The listing builds one solid part. Answer for the finished solid, in the listing's coordinates (mm). Coordinates: 2 decimals unless noted, no trailing zeros. Loops run counter-clockwise (first coordinate to the right, second up) from the corner with the lowest first, then second, coordinate; pieces in that order, holes last. Notation, with made-up numbers: M 52,61 L 75,61 A24 ccw 75,79 Z; hole C -33.75,-5.75 d3. An arc over 180 degrees is marked long. Answer as CSV lines item,"result". Start each with the question number.
```python
from build123d import *

# Parameters (mm, degrees)
SKETCH1_R                = 6.35
SKETCH1_R_2              = 2.159
BOSS_EXTRUDE1_DEPTH      = 5.0038
SKETCH6_R                = 9.715843696
SKETCH6_R_2              = 2.159
BOSS_EXTRUDE3_DEPTH      = 0.254
BOSS_EXTRUDE3_DEPTH_BACK = 5.0038
SKETCH2_R                = 2.159
CUT_EXTRUDE1_DEPTH       = 19.812


with BuildPart() as part:
    # Sketch1 → Boss-Extrude1 (new body)
    with BuildSketch(Plane.XY):
        with BuildLine():
            Line((-101.6, 12.7), (127, 12.7))
            ThreePointArc((127, 12.7), (139.7, 0), (127, -12.7))
            Line((127, -12.7), (-101.6, -12.7))
            ThreePointArc((-101.6, -12.7), (-114.3, 0), (-101.6, 12.7))
        make_face()
        with Locations((127, 0)):
            Circle(SKETCH1_R, mode=Mode.SUBTRACT)
        with Locations((-101.6, 0)):
            Circle(SKETCH1_R_2, mode=Mode.SUBTRACT)
    extrude(amount=BOSS_EXTRUDE1_DEPTH)

    # Sketch6 → Boss-Extrude3 (add, two sides)
    with BuildSketch(Plane.XY.offset(5.0038)) as boss_extrude3_sk:
        with Locations((127, 0)):
            Circle(SKETCH6_R)
        with Locations((127, 0)):
            Circle(SKETCH6_R_2, mode=Mode.SUBTRACT)
    extrude(amount=BOSS_EXTRUDE3_DEPTH)
    extrude(boss_extrude3_sk.sketch, amount=-BOSS_EXTRUDE3_DEPTH_BACK)

    # Sketch2 → Cut-Extrude1 (cut)
    with BuildSketch(Plane.XY.offset(5.0038)):
        Circle(SKETCH2_R)
    extrude(amount=-CUT_EXTRUDE1_DEPTH, mode=Mode.SUBTRACT)


solid = part.part
```
Item 1: Section D-D on x = 32.5 is taken. Determine the outline of the cut face in (y, z), then the cut area to 3 significant figures.
Item 2: For a pull along Y with two mould halves and no side action, classify faces 1 (the face through (129, -2, 5.258)), 2 (the face through (-99.54, 0.65, 2.47)), 3 (the face through (139.697, 0.279, 2.467)), 4 (the face through (-0.28, 2.14, 2.54)) as pulls with the +Y half, pulls with the -Y half, needs draft (parallel to the pull), parting line crosses it, or undercut.
Item 3: Section B-B on y = 0 is taken. Determine the outline of the cut face in (x, z), then the cut area to 3 significant figures.
Item 4: Section C-C on z = 2.45 is taken. Determine the outline of the cut face in (x, y).
Item 5: Section A-A on x = 0 is taken. Determine the outline of the cut face in (y, z).
Item 6: Consider line 1 (Y direction, x = -101.6, z = 3.45); line 2 (X direction, y = -1.25, z = 0.65); line 3 (X direction, y = -1.5, z = 3.8). Determine where each line is inside the solid, lowest interval first.
Item 7: Each of these flat-tipped pins is pushed along its axis until it touches: P1, Ø12.5, axis at x = 63, y = 6, coming from the +Z side; P2, Ø3, axis at y = 6.5, z = 3, coming from the -X side; P3, Ø3, axis at y = 8.5, z = 2, coming from the -X side. Where does it stop, or does it pass through?
Results are:
1,outline,"M -12.7,0 L 12.7,0 L 12.7,5 L -12.7,5 Z"
1,area,"127 mm²"
2,face 1,"needs draft"
2,face 2,"undercut"
2,face 3,"parting line crosses it"
2,face 4,"undercut"
3,outline,"M -114.3,0 L -103.76,0 L -103.76,5 L -114.3,5 Z; M -99.44,0 L -2.16,0 L -2.16,5 L -99.44,5 Z; M 2.16,0 L 124.84,0 L 124.84,5.26 L 117.28,5.26 L 117.28,5 L 2.16,5 Z; M 129.16,0 L 139.7,0 L 139.7,5 L 136.72,5 L 136.72,5.26 L 129.16,5.26 Z"
3,area,"1,210 mm²"
4,outline,"M -101.6,-12.7 L 127,-12.7 A12.7 ccw 127,12.7 L -101.6,12.7 A12.7 ccw Z; hole C -101.6,0 d4.32; hole C 0,0 d4.32; hole C 127,0 d4.32"
5,outline,"M -12.7,0 L -2.16,0 L -2.16,5 L -12.7,5 Z; M 2.16,0 L 12.7,0 L 12.7,5 L 2.16,5 Z"
6,line 1,"-12.7 to -2.16, 2.16 to 12.7"
6,line 2,"-114.24 to -103.36, -99.84 to -1.76, 1.76 to 125.24, 128.76 to 139.64"
6,line 3,"-114.21 to -103.15, -100.05 to -1.55, 1.55 to 125.45, 128.55 to 139.61"
7,P1,"z = 5"
7,P2,"x = -113.27"
7,P3,"x = -112.2"
